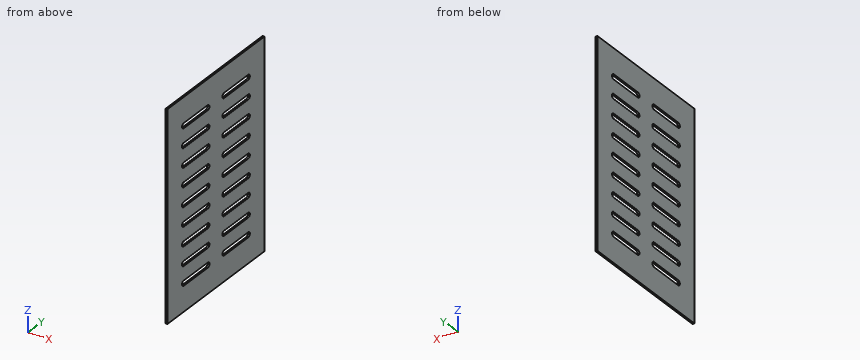
```python
from build123d import *

# Parameters (mm, degrees)
IZIM1_W                     = 330
IZIM1_H                     = 240
Y_KSEKLIK_EKSTR_ZYON1_DEPTH = 3


with BuildPart() as part:
    # Çizim1 → Yükseklik-Ekstrüzyon1 (new body)
    with BuildSketch(Plane(origin=(0, 0, 0), x_dir=(0, 0, -1), z_dir=(1, 0, 0))):
        with Locations((165, -120)):
            Rectangle(IZIM1_W, IZIM1_H)
        with BuildLine():
            Line((48, -40), (48, -100))
            ThreePointArc((48, -100), (44, -104), (40, -100))
            Line((40, -100), (40, -40))
            ThreePointArc((40, -40), (44, -36), (48, -40))
        make_face(mode=Mode.SUBTRACT)
        with BuildLine():
            Line((78.25, -40), (78.25, -100))
            ThreePointArc((78.25, -100), (74.25, -104), (70.25, -100))
            Line((70.25, -100), (70.25, -40))
            ThreePointArc((70.25, -40), (74.25, -36), (78.25, -40))
        make_face(mode=Mode.SUBTRACT)
        with BuildLine():
            Line((108.5, -40), (108.5, -100))
            ThreePointArc((108.5, -100), (104.5, -104), (100.5, -100))
            Line((100.5, -100), (100.5, -40))
            ThreePointArc((100.5, -40), (104.5, -36), (108.5, -40))
        make_face(mode=Mode.SUBTRACT)
        with BuildLine():
            Line((138.75, -40), (138.75, -100))
            ThreePointArc((138.75, -100), (134.75, -104), (130.75, -100))
            Line((130.75, -100), (130.75, -40))
            ThreePointArc((130.75, -40), (134.75, -36), (138.75, -40))
        make_face(mode=Mode.SUBTRACT)
        with BuildLine():
            Line((169, -40), (169, -100))
            ThreePointArc((169, -100), (165, -104), (161, -100))
            Line((161, -100), (161, -40))
            ThreePointArc((161, -40), (165, -36), (169, -40))
        make_face(mode=Mode.SUBTRACT)
        with BuildLine():
            Line((199.25, -40), (199.25, -100))
            ThreePointArc((199.25, -100), (195.25, -104), (191.25, -100))
            Line((191.25, -100), (191.25, -40))
            ThreePointArc((191.25, -40), (195.25, -36), (199.25, -40))
        make_face(mode=Mode.SUBTRACT)
        with BuildLine():
            Line((229.5, -40), (229.5, -100))
            ThreePointArc((229.5, -100), (225.5, -104), (221.5, -100))
            Line((221.5, -100), (221.5, -40))
            ThreePointArc((221.5, -40), (225.5, -36), (229.5, -40))
        make_face(mode=Mode.SUBTRACT)
        with BuildLine():
            Line((259.75, -40), (259.75, -100))
            ThreePointArc((259.75, -100), (255.75, -104), (251.75, -100))
            Line((251.75, -100), (251.75, -40))
            ThreePointArc((251.75, -40), (255.75, -36), (259.75, -40))
        make_face(mode=Mode.SUBTRACT)
        with BuildLine():
            Line((290, -40), (290, -100))
            ThreePointArc((290, -100), (286, -104), (282, -100))
            Line((282, -100), (282, -40))
            ThreePointArc((282, -40), (286, -36), (290, -40))
        make_face(mode=Mode.SUBTRACT)
        with BuildLine():
            Line((78.25, -140), (78.25, -200))
            ThreePointArc((78.25, -200), (74.25, -204), (70.25, -200))
            Line((70.25, -200), (70.25, -140))
            ThreePointArc((70.25, -140), (74.25, -136), (78.25, -140))
        make_face(mode=Mode.SUBTRACT)
        with BuildLine():
            Line((108.5, -140), (108.5, -200))
            ThreePointArc((108.5, -200), (104.5, -204), (100.5, -200))
            Line((100.5, -200), (100.5, -140))
            ThreePointArc((100.5, -140), (104.5, -136), (108.5, -140))
        make_face(mode=Mode.SUBTRACT)
        with BuildLine():
            Line((138.75, -140), (138.75, -200))
            ThreePointArc((138.75, -200), (134.75, -204), (130.75, -200))
            Line((130.75, -200), (130.75, -140))
            ThreePointArc((130.75, -140), (134.75, -136), (138.75, -140))
        make_face(mode=Mode.SUBTRACT)
        with BuildLine():
            Line((169, -140), (169, -200))
            ThreePointArc((169, -200), (165, -204), (161, -200))
            Line((161, -200), (161, -140))
            ThreePointArc((161, -140), (165, -136), (169, -140))
        make_face(mode=Mode.SUBTRACT)
        with BuildLine():
            Line((199.25, -140), (199.25, -200))
            ThreePointArc((199.25, -200), (195.25, -204), (191.25, -200))
            Line((191.25, -200), (191.25, -140))
            ThreePointArc((191.25, -140), (195.25, -136), (199.25, -140))
        make_face(mode=Mode.SUBTRACT)
        with BuildLine():
            Line((229.5, -140), (229.5, -200))
            ThreePointArc((229.5, -200), (225.5, -204), (221.5, -200))
            Line((221.5, -200), (221.5, -140))
            ThreePointArc((221.5, -140), (225.5, -136), (229.5, -140))
        make_face(mode=Mode.SUBTRACT)
        with BuildLine():
            Line((259.75, -140), (259.75, -200))
            ThreePointArc((259.75, -200), (255.75, -204), (251.75, -200))
            Line((251.75, -200), (251.75, -140))
            ThreePointArc((251.75, -140), (255.75, -136), (259.75, -140))
        make_face(mode=Mode.SUBTRACT)
        with BuildLine():
            Line((290, -140), (290, -200))
            ThreePointArc((290, -200), (286, -204), (282, -200))
            Line((282, -200), (282, -140))
            ThreePointArc((282, -140), (286, -136), (290, -140))
        make_face(mode=Mode.SUBTRACT)
        with BuildLine():
            Line((48, -140), (48, -200))
            ThreePointArc((48, -200), (44, -204), (40, -200))
            Line((40, -200), (40, -140))
            ThreePointArc((40, -140), (44, -136), (48, -140))
        make_face(mode=Mode.SUBTRACT)
    extrude(amount=Y_KSEKLIK_EKSTR_ZYON1_DEPTH)


solid = part.part
```
Here's how the part is built. I have some questions about the finished solid (model axes, mm). Give positions to 0.01 mm unless a question says otherwise; leave off trailing zeros. Write each loop counter-clockwise with the first axis right and the second up, starting at its lowest first coordinate (ties: lowest second). Pieces come first, ordered by that corner, then holes. Notation, with made-up numbers: M 43.25,67.25 L 92.25,67.25 A8 ccw 92.25,78.25 Z; hole C -6.75,-4.5 d7. An arc over 180 degrees is marked long. Put each result on its own line as item: value. Start each with the question number.
Item 1: Will this pin go through, and if not, where does the flat tip stop? pin 1 (1 mm diameter, centred on y = -94.5, z = -248, fed in from -X).
Item 2: If we section it at A-A, the plane z = -255.75: Write out the boundary of the cut face in (x, y).
Item 3: I need wall thicknesses on L1, parallel to Y at x = 0.9, z = -105; L2, parallel to Y at x = 1.9, z = -161.5. Which ranges of each line are inside material? Lowest first, please. Write a range as from..to.
Item 4: If we section it at B-B, the plane y = -45: Count the separate pieces of the cut face and the enclosed holes in it, then the cut area to 3 significant figures.
Values:
1. pin 1: x = 0
2. outline: M 0,-240 L 3,-240 L 3,-204 L 0,-204 Z; M 0,-136 L 3,-136 L 3,-104 L 0,-104 Z; M 0,-36 L 3,-36 L 3,0 L 0,0 Z
3. L1: -240..-203.97, -136.03..-103.97, -36.03..0
3. L2: -240..-201.94, -138.06..-101.94, -38.06..0
4. separate pieces: 10
4. enclosed holes: 0
4. area: 774 mm²
